Input: part model. Units: mm. Frame: model coordinates. A direction names the side the tool comes from. Coordinates: 2 decimals unless noted, no trailing zeros. Order: outer loops, then holes, each group sorted by start corner. A loop starts at its lowest first (then second) coordinate and runs counter-clockwise, first axis right, second up. Notation, with made-up numbers: (24, 8.5) -> (34, 8.5) arc R27 cw to (34, 46.5) -> close; hole circle Ø1 at (-17, 46.5). An arc over 180 degrees is marked (long way). Answer as CSV lines item,"result".
Autodesk Inventor part; units mm, degrees
ref_plane "Work Plane1" through (29, 0, 0) normal (0, -1, 0) x (1, 0, 0)
ref_plane "YZ Plane" through (0, 0, 0) normal (1, 0, 0) x (0, 1, 0)
ref_plane "XZ Plane" through (0, 0, 0) normal (0, 1, 0) x (-1, 0, 0)
sketch "Sketch1" plane through (0, 0, 0) normal (0, 0, 1) x (1, 0, 0)
  line L0 (0.2879, 0) -> (12.7, 0)
  line L1 (12.7, 0) -> (12.7, 2.413)
  line L2 (12.7, 2.413) -> (1.5878, 2.413)
  line L3 (1.5878, 2.413) -> (0.0002, 2.413)
  line L4 (0.0002, 2.413) -> (0, 2.413)
  line L5 (0, 2.413) -> (0, 4.5847)
  line L6 (0, 4.5847) -> (-2.5654, 4.5847)
  line L7 (-2.5654, 4.5847) -> (-2.5654, 1.8624)
  line L8 (-2.5654, 1.8624) -> (-0.7874, 1.8624)
  line L9 (-0.7874, 1.8624) -> (0.2879, 0)
  line L10 (-5.6185, 0) -> (15.7531, 0)
  line L11 (0, -0.9169) -> (0, 5.5016)
  line L12 (1.5878, 2.413) -> (0, 2.413) construction
  dimension "d1" = 11.1122
  dimension "d2" = 1.5876
  dimension "d3" = 2.5654
  dimension "d4" = 1.778
  dimension "d5" = 60
  dimension "d6" = 4.826
  dimension "d7" = 4.826
  dimension "d8" = 3.7248
  dimension "d9" = 9.1694
  dimension "d26" = 12.7
revolve "Body" add sketch "Sketch1" angle 360 about axis through (0.2879, 0, 0) along (1, 0, 0) contours L9 L11 L3 L2 L1 L0 | L9 L8 L7 L6 L5 L11
sketch "Sketch2" plane through (-2.5654, 0, 0) normal (-1, 0, 0) x (0, 0, 1)
  circle A0 centre (0, 0) radius 1.8624
  line L0 (0, -6.4186) -> (0, 6.4186)
  line L1 (-6.4186, 0) -> (6.4186, 0)
  line L2 (1.8624, 0) -> (0.9312, -1.6129)
  line L3 (0.9312, -1.6129) -> (-0.9312, -1.6129)
  line L4 (-0.9312, -1.6129) -> (-1.8624, 0)
  line L5 (-1.8624, 0) -> (-0.9312, 1.6129)
  line L6 (-0.9312, 1.6129) -> (0.9312, 1.6129)
  line L7 (0.9312, 1.6129) -> (1.8624, 0)
extrude "Slot" add sketch "Sketch2" against normal up to next contours L7 A0 | A0 L2 | L6 L0 A0 | A0 L0 L3 | L0 L6 A0 | A0 L3 L0 | L4 A0 | A0 L5
fillet "Fillet1" radius 1.778 1 edges at (-2.5654, -4.5847, 0)
thread "Thread"
chamfer "Chamfer1" distance 0.4869 distance2 0.4869 1 edges at (12.7, -2.413, 0) measured on face at (12.7, -0.2852, -0.7521)
ref_plane "Work Plane1" through (29, 0, 0) normal (0, -1, 0) x (1, 0, 0)
fillet "Fillet2" radius 0.1 1 edges at (0.0002, -2.413, 0)
equation "\"d30\" = R"
equation "\"d17\" = RR"
equation "\"d13\" = GEL"
equation "\"d15\" = -0.5 * SPD + 0.5 * GD"
equation "\"d16\" = GUL"
equation "\"d1\" = GEL"
equation "\"d3\" = KOH"
equation "\"d4\" = INTI"
equation "\"d6\" = GD"
equation "\"d7\" = BDM"
equation "\"d8\" = 1.1547 * SW"
equation "\"d9\" = KOD"
equation "\"d26\" = NLG"
equation "\"GD\" = NND"
equation "\"NLG\" = 12.7"
equation "\"GEL\" = 11.11225"
equation "\"KOD\" = 9.1694"
equation "\"KOH\" = 2.5654"
equation "\"INTI\" = 1.778"
equation "\"GAL\" = 1.5875"
equation "\"GUL\" = 0.48692"
equation "\"BDM\" = NND"
equation "\"SW\" = 3.2258"
equation "\"RR\" = 1.778"
equation "\"SPD\" = GD1"
equation "\"R\" = 0.1"
equation "\"KR\" = 4.699"
equation "\"GD1\" = 3.85216"
equation "\"THREADDIA\" = 4.826"
equation "\"FAWI\" = 45deg"
equation "\"KOH1\" = 1.778"
equation "\"NND\" = 4.826"
equation "\"TOA\" = 30deg"
equation "\"E0\" = 1.155 * SW"
properties part number "Unbrako - 10 x 1/2" material "Steel, Mild"
1. Ray query, line 1 along X through (y, z) = (-2.5, -0.25); line 2 along X through (y, z) = (0.5, -3.5); line 3 along Z through (x, y) = (7, 0). Return the intervals inside material, ascending.
Findings:
line 1,"x = -2.57 to 0"
line 2,"x = -2.41 to 0"
line 3,"z = -2.41 to 2.41"
2. Reachability of faces 4 (the face through (-2.565, -2, 0)), 5 (the face through (0, 3, -1)), 6 (the face through (-1.6, -0.8, -1.4)) from +Z, -Z, +X, -X, +Y, -Y: full face, straight path, thin tool, end or side. Return the list, or none.
Findings:
face 4,"+Z, -Z, -X, +Y, -Y"
face 5,"+X"
face 6,"-X"
3. Cut plane A-A (x = 2.75). Return the cut outline in (y, z), plus the area to 3 significant figures.
Findings:
outline,"circle Ø4.83 at (0, 0)"
area,"18.3 mm2"
4. Mould query, pull axis Z, two halves, no side actions, for faces 1 (the face through (12.7, 0, 0)), 2 (the face through (-2, -1.613, 0)), 3 (the face through (6.072, -1.915, 1.468)). Classes: released by +Z, released by -Z, zero draft, split by the parting line, or undercut.
Findings:
face 1,"zero draft"
face 2,"undercut"
face 3,"split by the parting line"
5. Contact query for flat-ended pins moving along their axis: pin 1 (1 mm diameter, centred on y = -3.5, z = 2.5, fed in from -X); pin 2 (1 mm diameter, centred on x = 1.5, y = -1.5, fed in from -Z); pin 3 (2 mm diameter, centred on x = -2, z = 0, fed in from -Y). Output: stop coordinate, or through.
Findings:
pin 1,"stops at x = -2.26"
pin 2,"stops at z = -2.2"
pin 3,"stops at y = -4.57"
